Could you check a few things on this model? Use its own coordinates, in mm. A direction names the side the tool comes from. Coordinates: 2 decimals unless noted, no trailing zeros. Loops run counter-clockwise (first coordinate to the right, second up) from the corner with the lowest first, then second, coordinate; pieces in that order, holes last. Notation, with made-up numbers: (-16.75, 27.5) - (8.25, 27.5) arc R24 cw to (8.25, 40.5) - close; hole circle Ø10 at (-31.5, -10). An arc over 180 degrees is marked (long way). One line per question, with ' | ' between items. Start each with the question number.
1. Which directions (+Z, -Z, +X, -X, +Y, -Y) give clear straight access to the entire face, cutting with the end or side of a thin tool? Please do faces 1 (the flat face through (2, 0.5, -25)), 2 (the flat face through (0, 8, -36)).
2. I want a section at C-C, the plane x = 3.35. Write out the boundary of the cut face in (y, z), then the cut area to 3 significant figures.
3. Please list where these lines run through material, in increasing order: L1, parallel to Z at x = 0.8, y = 11.75; L2, parallel to Y at x = 3.95, z = -23. Write a range as [from, to].
4. We'd pull the mould along Z, two halves only. Please class faces 3 (the flat face through (2, 7, -50)), 4 (the flat face through (2, 0, -25)), 5 (the flat face through (2, 7, -18)): pulls with the +Z half, pulls with the -Z half, needs draft (parallel to the pull), parting line crosses it, or undercut.
5. I want a section at A-A, the plane y = 10. Write out the boundary of the cut face in (x, z).
6. I want a section at B-B, the plane z = -23.5. Write out the boundary of the cut face in (x, y), then the cut area to 3 significant figures.
from build123d import *

# Parameters (mm, degrees)
SKETCH1_W           = 14
SKETCH1_H           = 14
BOSS_EXTRUDE1_DEPTH = 5


with BuildPart() as part:
    # Sketch1 → Boss-Extrude1 (new body)
    with BuildSketch(Plane(origin=(0, 0, 0), x_dir=(0, 0, -1), z_dir=(1, 0, 0))):
        Polygon((50, 15), (18, 15), (0, 15), (0, 0), (50, 0), align=None)
        with Locations((25, 7.5)):
            Rectangle(SKETCH1_W, SKETCH1_H, mode=Mode.SUBTRACT)
    extrude(amount=BOSS_EXTRUDE1_DEPTH)


solid = part.part
Results are:
1) face 1: +X, -X | face 2: +Z, -Z, -X, +Y, -Y
2) outline: (0, -50) - (15, -50) - (15, 0) - (0, 0) - close; hole (0.5, -32) - (14.5, -32) - (14.5, -18) - (0.5, -18) - close | area: 554 mm2
3) L1: z = [-50, -32], [-18, 0] | L2: y = [0, 0.5], [14.5, 15]
4) face 3: pulls with the -Z half | face 4: needs draft | face 5: undercut
5) outline: (0, -50) - (5, -50) - (5, -32) - (0, -32) - close; (0, -18) - (5, -18) - (5, 0) - (0, 0) - close
6) outline: (0, 0) - (5, 0) - (5, 0.5) - (0, 0.5) - close; (0, 14.5) - (5, 14.5) - (5, 15) - (0, 15) - close | area: 5.00 mm2
